Design review of the part built by this model. Coordinates are the model's own, in mm. A direction names the side the tool comes from. Coordinates: 2 decimals unless noted, no trailing zeros. Loops run counter-clockwise (first coordinate to the right, second up) from the corner with the lowest first, then second, coordinate; pieces in that order, holes last. Notation, with made-up numbers: (50, 5) - (75, 5) arc R18 cw to (75, 36) - close; hole circle Ø10 at (60.25, 81.25). An arc over 180 degrees is marked (long way). Answer in a Markdown table with one row per item. Add a question column.
(1) We need section C-C, the plane y = -3. Write out the cut boundary in (x, z), plus the area to 3 significant figures.
(2) For faces 4 (the face through (-1.67, -0.487, 12.716)), 5 (the face through (-1.86, -5.71, 14.18)), list the 3-axis set-ups (+Z, -Z, +X, -X, +Y, -Y) from which the entire face can be reached by the end or side of a thin tool; tool diameter is ignored.
(3) To check wall thickness, follow L1, parallel to Z at x = 0, y = -0.6 (3 decimals); L2, parallel to X at y = -3.75, z = 3.25; L3, parallel to Z at x = -10.75, y = -1.5. State the ranges of each line that lie inside material, in increasing order. Write a range as [from, to].
(4) We need section A-A, the plane x = 0. Write out the cut boundary in (y, z) (3 decimals).
(5) We need section D-D, the plane y = -0.5. Write out the cut boundary in (x, z) (3 decimals).
(6) Clearance check with flat-ended pins moving along their axes: pin 1 (10 mm diameter, centred on x = -9, z = -1, fed in from -Y); pin 2 (1.5 mm diameter, centred on y = -5.5, z = 4.5, fed in from -X). State where each tip first meets the part, or that it passes through.
(7) The part is to be moulded in two halves that separate along Z. For faces 1 (the face through (11, 0, 7)), 2 (the face through (-14.985, -3.18, 0.66)), 3 (the face through (13.277, -3.086, 2.948)), say which applies: released by +Z, released by -Z, zero draft, split by the parting line, or undercut.
(8) We need section B-B, the plane z = 0. Write out the cut boundary in (x, y) (3 decimals), plus the area to 3 significant figures.
from build123d import *

# Parameters (mm, degrees)
F0_R     = 15
F0_R_2   = 12.825
F1_DEPTH = 6.45
F2_R     = 14.3
F3_DEPTH = 1.5
F4_R     = 14.1
F5_DEPTH = 1.4


with BuildPart() as f1:
    # F0 (on Front) → F1 (new body)
    with BuildSketch(Plane.XZ):
        Circle(F0_R)
        Circle(F0_R_2, mode=Mode.SUBTRACT)
    extrude(amount=F1_DEPTH)

    # F2 (on face) → F3 (cut)
    with BuildSketch(Plane.XZ.offset(6.45)):
        Circle(F2_R)
    extrude(amount=-F3_DEPTH, mode=Mode.SUBTRACT)

    # F4 (on face) → F5 (cut)
    with BuildSketch(Plane.XZ.offset(4.95)):
        Circle(F4_R)
    extrude(amount=-F5_DEPTH, mode=Mode.SUBTRACT)

    # F6 (on Right) → F7 (revolve, cut)
    with BuildSketch(Plane.YZ):
        with BuildLine():
            ThreePointArc((-2.634126, -13.6), (-1.125071, -12.974929), (-0.5, -11.465874))
            Line((-0.5, -11.465874), (-0.5, 0))
            Line((-0.5, 0), (-3.55, 0))
            Line((-3.55, 0), (-3.55, -13.6))
            Line((-3.55, -13.6), (-2.634126, -13.6))
        make_face()
    revolve(axis=Axis((0, -2.025, 0), (0, 1, 0)), mode=Mode.SUBTRACT)


solid = f1.part
Responses:
| question | item | result |
|---|---|---|
| 1 | outline | circle Ø30 at (0, 0); hole circle Ø27.2 at (0, 0) |
| 1 | area | 126 mm2 |
| 2 | face 4 | +Y, -Y |
| 2 | face 5 | -Y |
| 3 | L1 | z = [-15, -12.825], [12.825, 15] |
| 3 | L2 | x = [-14.64, -13.72], [13.72, 14.64] |
| 3 | L3 | z = [-10.46, -7.79], [7.79, 10.46] |
| 4 | outline | (-6.45, -15) - (0, -15) - (0, -12.825) - (-0.989, -12.825) arc R2.134 cw to (-2.634, -13.6) - (-3.55, -13.6) - (-3.55, -14.1) - (-4.95, -14.1) - (-4.95, -14.3) - (-6.45, -14.3) - close; (-6.45, 14.3) - (-4.95, 14.3) - (-4.95, 14.1) - (-3.55, 14.1) - (-3.55, 13.6) - (-2.634, 13.6) arc R2.134 cw to (-0.989, 12.825) - (0, 12.825) - (0, 15) - (-6.45, 15) - close |
| 5 | outline | circle Ø30 at (0, 0); hole circle Ø25.65 at (0, 0) |
| 6 | pin 1 | stops at y = -3.55 |
| 6 | pin 2 | stops at x = -14.52 |
| 7 | face 1 | zero draft |
| 7 | face 2 | split by the parting line |
| 7 | face 3 | undercut |
| 8 | outline | (-15, -6.45) - (-14.3, -6.45) - (-14.3, -4.95) - (-14.1, -4.95) - (-14.1, -3.55) - (-13.6, -3.55) - (-13.6, -2.634) arc R2.134 cw to (-12.825, -0.989) - (-12.825, 0) - (-15, 0) - close; (12.825, -0.989) arc R2.134 cw to (13.6, -2.634) - (13.6, -3.55) - (14.1, -3.55) - (14.1, -4.95) - (14.3, -4.95) - (14.3, -6.45) - (15, -6.45) - (15, 0) - (12.825, 0) - close |
| 8 | area | 16.9 mm2 |
